Verification items for the finished model (mm, model axes). A direction names the side the tool comes from. Give positions to 0.01 mm unless a question says otherwise; leave off trailing zeros. Write each loop counter-clockwise with the first axis right and the second up, starting at its lowest first coordinate (ties: lowest second). Pieces come first, ordered by that corner, then holes. Notation, with made-up numbers: M 45,6 L 79,6 A20 cw 79,40 Z; hole C -10,81.5 d8. An arc over 180 degrees is marked long. Write item = value, one per line.
from build123d import *

# Parameters (mm, degrees)
F1_DEPTH = 22.225
F2_R     = 5.5118
F3_DEPTH = 17.78
F5_D     = 9.1186


# Not quite as in the source:
# - ends of sketch curves that miss each other by under 0.0002 mm in the source are joined


with BuildPart() as f1:
    # F0 (on Front) → F1 (new body)
    with BuildSketch(Plane.XZ):
        with BuildLine():
            ThreePointArc((7.0042338121, -8.6271875461), (10.9449391879, -1.9224886016), (9.5250001177, 5.7238124539))
            Line((9.5250001177, 5.7238124539), (-9.5250001177, 5.7238124539))
            ThreePointArc((-9.5250001177, 5.7238124539), (-10.9449391879, -1.9224886016), (-7.0042338121, -8.6271875461))
            Line((-7.0042338121, -8.6271875461), (7.0042338121, -8.6271875461))
        make_face()
    extrude(amount=F1_DEPTH)

    # F2 (on face) → F3 (join)
    with BuildSketch(Plane.XZ.offset(22.225)):
        Circle(F2_R)
    extrude(amount=F3_DEPTH)

    # F5 (through all)
    with Locations(Plane(origin=(0, 0, -8.6271875461), x_dir=(1, 0, 0), z_dir=(0, 0, -1))):
        with Locations((0, 11.43)):
            Hole(F5_D / 2)


solid = f1.part
1) Tool access check on faces 4 (the flat face through (0, -40.005, 0)), 5 (the cylindrical face through (-1.19, -30.99, -5.38)). Record the directions out of +Z, -Z, +X, -X, +Y, -Y that give a thin tool (end or side, any length) a straight path to the whole face; none if there is none.
From the geometry:
face_4 = +Z, -Z, +X, -X, -Y
face_5 = -Y
2) Cross-section at D-D on y = -28. Record the boundary of the cut face in (x, z).
From the geometry:
outline = C 0,0 d11.02
3) Draft check along X on faces 1 (the cylindrical face through (10.925, -10.957, -2.032)), 2 (the flat face through (0, -22.225, -6)), 3 (the cylindrical face through (0.99, -6.98, -1.35)). Enter one of: +X half, -X half, draft (parallel to the pull), parting line (faces both ways), or undercut.
From the geometry:
face_1 = +X half
face_2 = draft
face_3 = undercut
4) Cross-section at A-A on x = 0. Record the boundary of the cut face in (y, z) (3 decimals), plus the area to 3 significant figures.
From the geometry:
outline = M -40.005,-5.512 L -22.225,-5.512 L -22.225,-8.627 L -15.989,-8.627 L -15.989,5.724 L -22.225,5.724 L -22.225,5.512 L -40.005,5.512 Z; M -6.871,-8.627 L 0,-8.627 L 0,5.724 L -6.871,5.724 Z
area = 384 mm^2
5) Cross-section at B-B on y = -11.43. Record the boundary of the cut face in (x, z) (1 decimal), plus the area to 3 significant figures.
From the geometry:
outline = M -9.5,5.7 A11.1 ccw -7,-8.6 L -4.6,-8.6 L -4.6,5.7 Z; M 4.6,-8.6 L 7,-8.6 A11.1 ccw 9.5,5.7 L 4.6,5.7 Z
area = 161 mm^2
6) Material ranges on probe 1 along Y at (x, z) = (0, -1.5) (3 decimals); probe 2 along Y at (x, z) = (-3.5, 4) (3 decimals); probe 3 along Y at (x, z) = (10, -3.75) (3 decimals), recorded low to high. Write a range as from..to.
From the geometry:
probe_1 = -40.005..-15.989, -6.871..0
probe_2 = -40.005..-14.352, -8.508..0
probe_3 = -22.225..0
7) Depth check by flat-ended pin: P1, Ø4, axis at y = -9.5, z = -5.5, coming from the +X side; P2, Ø3, axis at y = -7.5, z = -1, coming from the +X side; P3, Ø1, axis at x = 3.5, y = -27.5, coming from the -Z side; P4, Ø8, axis at x = 4, y = -34.5, coming from the +Z side. Enter the tip coordinate at first touch or a pass-through.
From the geometry:
P1 = 10.55
P2 = 11.11
P3 = -4.62
P4 = 5.51
8) Cross-section at C-C on z = 0. Record the boundary of the cut face in (x, y) (1 decimal), plus the area to 3 significant figures.
From the geometry:
outline = M -11.1,-22.2 L -5.5,-22.2 L -5.5,-40 L 5.5,-40 L 5.5,-22.2 L 11.1,-22.2 L 11.1,0 L -11.1,0 Z; hole C 0,-11.4 d9.1
area = 625 mm^2
